CAD build for the part. Positions are in the model's coordinates, mm. A direction names the side the tool comes from. Round coordinates to 2 decimals unless told otherwise and drop trailing zeros. Write each loop counter-clockwise with the first axis right and the second up, starting at its lowest first coordinate (ties: lowest second). Pieces come first, ordered by that corner, then holes. Notation, with made-up numbers: (-37.75, 23) - (-28.75, 23) arc R18 cw to (-28.75, 36) - close; hole circle Ø9 at (-20.75, 45). An arc over 180 degrees is marked (long way). Use one line per item in the form item = value. Start each with the question number.
Item 1: Band-saw the part on A-A, the plane x = 1. List the corners of the cut face in (y, z), and give its area (3 significant figures).
Item 2: Drill centre lines: L1, parallel to X at y = 4.75, z = 1; L2, parallel to Z at x = 3.75, y = 0.5; L3, parallel to Y at x = 5.75, z = 1.25. Where is each one in solid material? Low to high.
Item 3: Tool access for faces 1 (the flat face through (-0.6, -7, 0)), 2 (the flat face through (-0.6, 7, 0)), 3 (the flat face through (-2.92, -5.66, -3.2)), 4 (the cylindrical face through (-0.296, -5.158, -3.955)): list every direction of +Z, -Z, +X, -X, +Y, -Y with a clear straight run to the whole face (end or side of a thin tool).
Item 4: Pin check, flat tips, straight feed: pin 1 (1.5 mm diameter, centred on y = -5, z = -4, fed in from +X); pin 2 (2 mm diameter, centred on x = 8, y = 3.5, fed in from -Z); pin 3 (6 mm diameter, centred on x = 9, y = -5, fed in from -Z). Stop position of each tip, or through.
Autodesk Inventor part; units mm, degrees
ref_plane "Work Plane1" through (1.525, 0, 0) normal (0, 0, 1) x (1, 0, 0)
ref_plane "YZ Plane" through (0, 0, 0) normal (1, 0, 0) x (0, 1, 0)
ref_plane "XZ Plane" through (0, 0, 0) normal (0, 1, 0) x (-1, 0, 0)
sketch "Sketch1" plane through (0, 0, 0) normal (0, 0, 1) x (1, 0, 0)
  line L0 (0, 6.5) -> (0, 4)
  line L1 (3.7, 4) -> (12, 4)
  line L2 (12, 4) -> (12, 0)
  line L3 (12, 0) -> (-0.6001, 0)
  line L4 (-3.1201, 0) -> (14.52, 0)
  line L5 (-0.6001, 0) -> (-0.6001, 6.5)
  line L6 (-0.6001, 6.5) -> (0, 6.5)
  line L7 (3.7, 4) -> (2.9331, 4)
  line L8 (2.9331, 4) -> (0, 4)
  line L9 (0, -1.3) -> (0, 7.8)
  dimension "d0" = 12
  dimension "d1" = 8.3
  dimension "d2" = 8
  dimension "d9" = 0.6001
  dimension "d10" = 13
  dimension "d13" = 0.7669
  dimension "d14" = 8
revolve "Body" add sketch "Sketch1" angle 360 about axis through (12, 0, 0) along (-1, 0, 0)
sketch "Sketch2" plane through (-0.6001, 0, 0) normal (-1, 0, 0) x (0, 0, 1)
  line L0 (0, 7.5056) -> (6.5, 3.7528)
  line L1 (6.5, 3.7528) -> (6.5, -3.7528)
  line L2 (6.5, -3.7528) -> (0, -7.5056)
  line L3 (0, -7.5056) -> (-6.5, -3.7528)
  line L4 (-6.5, -3.7528) -> (-6.5, 3.7528)
  line L5 (-6.5, 3.7528) -> (0, 7.5056)
  point P0 (0, 0)
  point P1 (0, 0)
  dimension "d11" = 13
extrude "Head" add sketch "Sketch2" along normal blind 4.7
sketch "Sketch4" plane through (0, 0, 0) normal (0, 0, 1) x (1, 0, 0)
  line L0 (-5.3001, 6.5) -> (-5.3001, 7.5056)
  line L1 (-5.3001, 7.5056) -> (-4.7195, 7.5056)
  line L2 (-4.7195, 7.5056) -> (-5.3001, 6.5)
  line L3 (-6.2401, 0) -> (0.3399, 0)
  line L4 (-0.6001, 7.5056) -> (-5.3001, 7.5056)
  line L5 (-5.3001, 3.7528) -> (-5.3001, 7.5056)
  dimension "d5" = 30
  dimension "d19" = 13
revolve "Chamfer1" cut sketch "Sketch4" angle 360 about axis through (-10, 0, 0) along (1, 0, 0)
thread "Thread"
chamfer "Chamfer2" distance 0.7668 distance2 0.7669 1 edges at (12, -4, 0) measured on face at (12, -0.0467, -2.2623)
ref_plane "Work Plane1" through (1.525, 0, 0) normal (0, 0, 1) x (1, 0, 0)
equation "\"d0\" = NLG"
equation "\"d1\" = GEL"
equation "\"d2\" = GD"
equation "\"d10\" = SD2"
equation "\"d14\" = BDM"
equation "\"d11\" = SW"
equation "\"d3\" = KOH - SD"
equation "\"d5\" = ANG1"
equation "\"d19\" = SW0"
equation "\"d15\" = GEL"
equation "\"d6\" = -0.5 * SPD + 0.5 * GD"
equation "\"NLG\" = 12"
equation "\"GD\" = NND"
equation "\"BDM\" = NND"
equation "\"KOH\" = 5.3"
equation "\"GEL\" = 8.3"
equation "\"SW\" = 13"
equation "\"SW0\" = SW"
equation "\"SPD\" = NND - 1.2269 * PTC"
equation "\"SD2\" = SW"
equation "\"SD\" = 0.6"
equation "\"ANG1\" = 30deg"
equation "\"GAL\" = 0.61345 * PTC"
equation "\"GUL\" = 0.61345 * PTC"
equation "\"RR\" = 0.4"
equation "\"WFT\" = SD"
equation "\"GD1\" = THREADDIA - 1.2269 * PTC"
equation "\"THREADDIA\" = 8"
equation "\"SDH\" = SW"
equation "\"TOA\" = 30deg"
equation "\"FAWI\" = 45deg"
equation "\"PTC\" = 1.25"
equation "\"NND\" = 8"
equation "\"E0\" = 1.155 * SW"
properties part number "AS 1110 - M8 x 12" material "Steel, Mild"
Determined:
q1.outline = circle Ø8 at (0, 0)
q1.area = 50.3 mm²
q2.L1 = -5.3 to 0
q2.L2 = -3.97 to 3.97
q2.L3 = -3.8 to 3.8
q3.face_1 = +X, -Y
q3.face_2 = +X, +Y
q3.face_3 = -Z, +X, -X, -Y
q3.face_4 = +X
q4.pin_1 = 0
q4.pin_2 = -3.12
q4.pin_3 = -3.46
